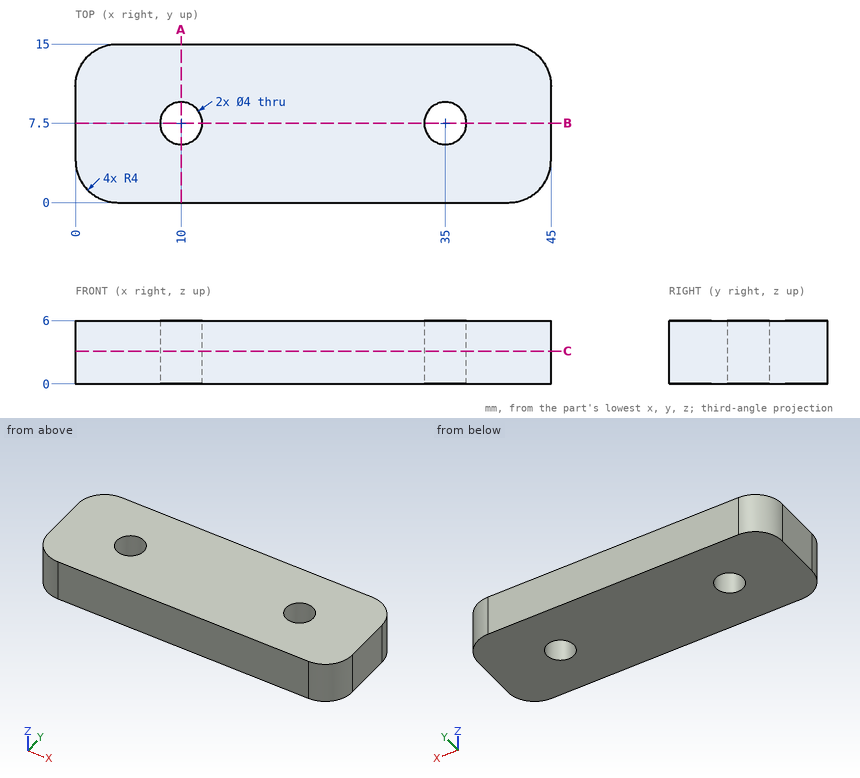
Study the drawing (mm; zero at the part's minimum x, y, z) and answer. Give positions to 0.01 mm unless a question says otherwise; leave off trailing zeros. Write each loop counter-clockwise with the first axis right and the second up, starting at its lowest first coordinate (ties: lowest second). Pieces come first, ordered by that corner, then holes. Notation, with made-up numbers: M -2.75,-36.75 L 13.25,-36.75 A12 cw 13.25,-17.75 Z; hole C -36.75,13 d7. An arc over 180 degrees is marked long. Put each result on its own line as item: value. Start each with the question number.
1. The part is cut by section A-A, the plane x = 10. Give the vertices of the cut face in (y, z), and give its area (3 significant figures).
2. Consider line 1 along X through (y, z) = (6.25, 2.25); line 2 along Y through (x, z) = (36.5, 4); line 3 along Y through (x, z) = (35, 4.05). Determine where each line is inside the solid, lowest interval first.
3. The part is cut by section C-C, the plane z = 3.1. Give the vertices of the cut face in (x, y).
4. The part is cut by section B-B, the plane y = 7.5. Give the vertices of the cut face in (x, z).
Final values:
1. outline: M 0,0 L 5.5,0 L 5.5,6 L 0,6 Z; M 9.5,0 L 15,0 L 15,6 L 9.5,6 Z
1. area: 66.0 mm²
2. line 1: x = 0 to 8.44, 11.56 to 33.44, 36.56 to 45
2. line 2: y = 0 to 6.18, 8.82 to 15
2. line 3: y = 0 to 5.5, 9.5 to 15
3. outline: M 0,4 A4 ccw 4,0 L 41,0 A4 ccw 45,4 L 45,11 A4 ccw 41,15 L 4,15 A4 ccw 0,11 Z; hole C 10,7.5 d4; hole C 35,7.5 d4
4. outline: M 0,0 L 8,0 L 8,6 L 0,6 Z; M 12,0 L 33,0 L 33,6 L 12,6 Z; M 37,0 L 45,0 L 45,6 L 37,6 Z
